Input: part model. Units: mm. Frame: model coordinates. A direction names the side the tool comes from. Coordinates: 2 decimals unless noted, no trailing zeros. Order: outer loops, then holes, each group sorted by start corner. A loop starts at its lowest first (then second) coordinate and runs counter-clockwise, first axis right, second up. Notation, with made-up numbers: (58.25, -5) - (63.25, -5) arc R20 cw to (63.25, 16) - close; hole circle Ø2 at (72, 37). An arc over 180 degrees is marked (long way). One line per question, with ' | ' between items. Start each with the question number.
```python
from build123d import *

# Parameters (mm, degrees)
F0_W      = 177.8
F0_H      = 101.6
F1_DEPTH  = 12.7
F2_R      = 3.175
F3_DEPTH  = 1.524
F4_R      = 1.5621
F5_DEPTH  = 6.35
F6_SIZE   = 0.762
F7_R      = 6.35
F8_R      = 1.5875
F9_DEPTH  = 12.701
F10_R     = 1.5875
F11_DEPTH = 12.701
F12_R     = 3.81
F13_DEPTH = 6.35
F15_DEPTH = 12.701
F17_DEPTH = 6.35
F18_R     = 1.5875
F19_DEPTH = 12.701
F20_R     = 3.81
F21_DEPTH = 6.35


with BuildPart() as f1:
    # F0 (on Top) → F1 (new body)
    with BuildSketch(Plane.XY):
        Rectangle(F0_W, F0_H)
    extrude(amount=F1_DEPTH)

    # F2 (on Top) → F3 (join)
    with BuildSketch(Plane.XY):
        with Locations((-38.1, 0)):
            Circle(F2_R)
        with Locations((38.1, 0)):
            Circle(F2_R)
        with Locations((0, -15.875)):
            Circle(F2_R)
    extrude(amount=-F3_DEPTH)

    # F4 (on face) → F5 (join)
    with BuildSketch(Plane(origin=(0, 0, -1.524), x_dir=(1, 0, 0), z_dir=(0, 0, -1))):
        with Locations((-38.1, 0)):
            Circle(F4_R)
        with Locations((38.1, 0)):
            Circle(F4_R)
        with Locations((0, 15.875)):
            Circle(F4_R)
    extrude(amount=F5_DEPTH)

    # F6
    f6_edges = [f1.edges().sort_by_distance(p)[0] for p in [
        (-39.6621, 0, -7.874),
        (-1.5621, -15.875, -7.874),
        (36.5379, 0, -7.874),
    ]]
    chamfer(f6_edges, length=F6_SIZE)

    # F7
    f7_edges = [f1.edges().sort_by_distance(p)[0] for p in [
        (-88.9, -50.8, 6.35),
        (88.9, -50.8, 6.35),
        (88.9, 50.8, 6.35),
        (-88.9, 50.8, 6.35),
    ]]
    fillet(f7_edges, radius=F7_R)

    # F8 (on face) → F9 (cut, through all)
    with BuildSketch(Plane(origin=(0, 0, 0), x_dir=(1, 0, 0), z_dir=(0, 0, -1))):
        with Locations((82.55, 44.45)):
            Circle(F8_R)
        with Locations((82.55, -44.45)):
            Circle(F8_R)
        with Locations((-82.55, -44.45)):
            Circle(F8_R)
        with Locations((-82.55, 44.45)):
            Circle(F8_R)
    extrude(amount=-F9_DEPTH, mode=Mode.SUBTRACT)

    # F10 (on face) → F11 (cut, through all)
    with BuildSketch(Plane(origin=(0, 0, 0), x_dir=(1, 0, 0), z_dir=(0, 0, -1))):
        with Locations((0, 31.75)):
            Circle(F10_R)
        with Locations((0, -31.75)):
            Circle(F10_R)
    extrude(amount=-F11_DEPTH, mode=Mode.SUBTRACT)

    # F12 (on face) → F13 (cut)
    with BuildSketch(Plane.XY.offset(12.7)):
        with Locations((0, 31.75)):
            Circle(F12_R)
        with Locations((0, -31.75)):
            Circle(F12_R)
    extrude(amount=-F13_DEPTH, mode=Mode.SUBTRACT)

    # F14 (on face) → F15 (cut, through all)
    with BuildSketch(Plane(origin=(0, 0, 0), x_dir=(1, 0, 0), z_dir=(0, 0, -1))):
        with BuildLine():
            ThreePointArc((16.637, 26.924), (13.081, 30.48), (9.525, 26.924))
            Line((9.525, 26.924), (9.525, -10.414))
            ThreePointArc((9.525, -10.414), (13.081, -13.97), (16.637, -10.414))
            Line((16.637, -10.414), (16.637, 26.924))
        make_face()
    extrude(amount=-F15_DEPTH, mode=Mode.SUBTRACT)

    # F16 (on face) → F17 (cut)
    with BuildSketch(Plane.XY.offset(12.7)):
        with BuildLine():
            Line((19.812, -26.924), (19.812, 10.414))
            ThreePointArc((19.812, 10.414), (13.081, 17.145), (6.35, 10.414))
            Line((6.35, 10.414), (6.35, -26.924))
            ThreePointArc((6.35, -26.924), (13.081, -33.655), (19.812, -26.924))
        make_face()
    extrude(amount=-F17_DEPTH, mode=Mode.SUBTRACT)

    # F18 (on face) → F19 (cut, through all)
    with BuildSketch(Plane(origin=(0, 0, 0), x_dir=(1, 0, 0), z_dir=(0, 0, -1))):
        with Locations((76.2, 0)):
            Circle(F18_R)
        with Locations((-76.2, 0)):
            Circle(F18_R)
    extrude(amount=-F19_DEPTH, mode=Mode.SUBTRACT)

    # F20 (on face) → F21 (cut)
    with BuildSketch(Plane.XY.offset(12.7)):
        with Locations((-76.2, 0)):
            Circle(F20_R)
        with Locations((76.2, 0)):
            Circle(F20_R)
    extrude(amount=-F21_DEPTH, mode=Mode.SUBTRACT)


solid = f1.part
```
(1) Reachability of faces 4 (the face through (-0.34, -14.35, -4.28)), 5 (the face through (-1, 50.8, 6)), 6 (the face through (19.812, -9, 10)), 7 (the face through (13, 13.97, 3.13)) from +Z, -Z, +X, -X, +Y, -Y: full face, straight path, thin tool, end or side. Return the list, or none.
(2) Material intervals for line 1 along X through (y, z) = (-44.45, 5); line 2 along Y through (x, z) = (0, 3.75); line 3 along Y through (x, z) = (-76.2, 10), sorted ascending. Write a range as from..to.
(3) Pin query (flat end, axial travel): pin 1 (6 mm diameter, centred on x = -77.5, y = 1.5, fed in from +Z); pin 2 (3.5 mm diameter, centred on x = -76.2, y = 0, fed in from +Z); pin 3 (5 mm diameter, centred on x = 0, y = 31.75, fed in from -Z). Return the tip coordinate at first contact, or that it passes through.
(4) Draft query along Y for faces 1 (the face through (-87.09, -48.89, 6.44)), 2 (the face through (-76, -2, 6.35)), 3 (the face through (39.5, -1.4, -1.524)). Return one class per face: +Y half, -Y half, draft (parallel to the pull), parting line (faces both ways), or undercut.
(5) Section A-A (z = 3.5). State how many separate pieces and enclosed holes the cut face has, then the cut area to 3 significant figures.
(6) Section B-B (x = -43.5). Output: boundary loops of the cut face in (y, z).
Worked answers:
1) face 4: -Z | face 5: +Z, -Z, +X, -X, +Y | face 6: +Z | face 7: +Z, -Z
2) line 1: x = -88.9..-84.14, -80.96..80.96, 84.14..88.9 | line 2: y = -50.8..-33.34, -30.16..30.16, 33.34..50.8 | line 3: y = -50.8..-3.81, 3.81..50.8
3) pin 1: stops at z = 12.7 | pin 2: stops at z = 6.35 | pin 3: stops at z = 0
4) face 1: -Y half | face 2: undercut | face 3: draft
5) separate pieces: 1 | enclosed holes: 9 | area: 17,700 mm²
6) outline: (-50.8, 0) - (50.8, 0) - (50.8, 12.7) - (-50.8, 12.7) - close
